```python
from build123d import *

# Parameters (mm, degrees)
BOSS_EXTRUDE1_DEPTH = 24
SKETCH2_R           = 10
BOSS_EXTRUDE2_DEPTH = 24
CIRPATTERN1_COUNT   = 4
BOSS_EXTRUDE4_START = -38
BOSS_EXTRUDE4_DEPTH = 14
BOSS_EXTRUDE5_DEPTH = 14
CUT_EXTRUDE1_DEPTH  = 102.434708064
FILLET1_R           = 10
FILLET2_R           = 10


with BuildPart() as part:
    # Sketch1 → Boss-Extrude1 (new body)
    with BuildSketch(Plane.YZ):
        with BuildLine():
            Line((81, 12), (81, 26))
            Line((81, 26), (37, 26))
            ThreePointArc((37, 26), (23.509262437, 22.226110771), (13.934874811, 12))
            Line((13.934874811, 12), (-37, 12))
            Line((-37, 12), (-37, -12))
            Line((-37, -12), (13.934874811, -12))
            ThreePointArc((13.934874811, -12), (23.509262437, -22.226110771), (37, -26))
            Line((37, -26), (81, -26))
            Line((81, -26), (81, -12))
            Line((81, -12), (37, -12))
            ThreePointArc((37, -12), (25, 0), (37, 12))
            Line((37, 12), (81, 12))
        make_face()
    extrude(amount=BOSS_EXTRUDE1_DEPTH)

    # Sketch2 → Boss-Extrude2 (add)
    with BuildSketch(Plane.XZ.offset(37)):
        with Locations(Location((12, 0, 0), (0, 0, 270))):
            Circle(SKETCH2_R)
    extrude(amount=BOSS_EXTRUDE2_DEPTH)

    # Sketch3 → Cut-Revolve2 (revolve, cut)
    with BuildSketch(Plane.YZ.offset(24)):
        with BuildLine():
            Line((-37, 12), (-37, 6))
            Line((-37, 6), (-17, 6))
            ThreePointArc((-17, 6), (-12.757359313, 7.757359313), (-11, 12))
            Line((-11, 12), (-37, 12))
        make_face()
    cut_revolve2 = revolve(axis=Axis((24, 13.934874811, 12), (0, 1, 0)), mode=Mode.SUBTRACT)

    # CirPattern1: Cut-Revolve2 ×4 about axis
    cirpattern1_axis = Axis((12, 0, 0), (0, 1, 0))
    for i in range(1, CIRPATTERN1_COUNT):
        add(cut_revolve2.rotate(cirpattern1_axis, i * 360 / CIRPATTERN1_COUNT), mode=Mode.SUBTRACT)

    # Sketch4 → Boss-Extrude4 (add, through all)
    with BuildSketch(Plane.XY.offset(26).offset(BOSS_EXTRUDE4_START)):
        with BuildLine():
            Line((24, 61), (24, 45))
            ThreePointArc((24, 45), (29.88854382, 52.05572809), (32, 61))
            ThreePointArc((32, 61), (29.88854382, 69.94427191), (24, 77))
            Line((24, 77), (24, 61))
        make_face()
        with BuildLine():
            Line((0, 45), (0, 61))
            Line((0, 61), (0, 77))
            ThreePointArc((0, 77), (-8, 61), (0, 45))
        make_face()
    extrude(amount=-BOSS_EXTRUDE4_DEPTH)

    # Sketch4<3> → Boss-Extrude5 (add)
    with BuildSketch(Plane.XY.offset(26)):
        with BuildLine():
            Line((24, 61), (24, 45))
            ThreePointArc((24, 45), (29.88854382, 52.05572809), (32, 61))
            ThreePointArc((32, 61), (29.88854382, 69.94427191), (24, 77))
            Line((24, 77), (24, 61))
        make_face()
        with BuildLine():
            Line((0, 45), (0, 61))
            Line((0, 61), (0, 77))
            ThreePointArc((0, 77), (-8, 61), (0, 45))
        make_face()
    extrude(amount=-BOSS_EXTRUDE5_DEPTH)

    # Sketch4<4> → Cut-Extrude1 (cut, through all)
    with BuildSketch(Plane.XY.offset(26)):
        with BuildLine():
            Line((24, 81), (12, 81))
            ThreePointArc((12, 81), (18.32455532, 79.973665961), (24, 77))
            Line((24, 77), (24, 81))
        make_face()
        with BuildLine():
            Line((0, 81), (0, 77))
            ThreePointArc((0, 77), (5.67544468, 79.973665961), (12, 81))
            Line((12, 81), (0, 81))
        make_face()
        with BuildLine():
            ThreePointArc((22, 61), (12, 71), (2, 61))
            Line((2, 61), (12, 61))
            Line((12, 61), (22, 61))
        make_face()
        with BuildLine():
            Line((12, 61), (2, 61))
            ThreePointArc((2, 61), (12, 51), (22, 61))
            Line((22, 61), (12, 61))
        make_face()
    extrude(amount=-CUT_EXTRUDE1_DEPTH, mode=Mode.SUBTRACT)

    # Fillet1
    fillet1_edges = [part.edges().sort_by_distance(p)[0] for p in [
        (24, 45, -19),
        (0, 45, -19),
        (24, 45, 19),
        (0, 45, 19),
    ]]
    fillet(fillet1_edges, radius=FILLET1_R)

    # Fillet2
    fillet2_edges = [part.edges().sort_by_distance(p)[0] for p in [
        (12, 13.934874811, -12),
        (12, 13.934874811, 12),
    ]]
    fillet(fillet2_edges, radius=FILLET2_R)


solid = part.part
```
Part model, mm, in its own coordinate system. A direction names the side the tool comes from. Coordinates: 2 decimals unless noted, no trailing zeros. Order: outer loops, then holes, each group sorted by start corner. A loop starts at its lowest first (then second) coordinate and runs counter-clockwise, first axis right, second up. Notation, with made-up numbers: (51.5, 49.25) - (67.5, 49.25) arc R19 ccw to (67.5, 78.25) - close; hole circle Ø2 at (59.25, 3.5). An arc over 180 degrees is marked (long way). Return JSON: item names as keys, results as strings. Group by question number.
Item 1: Cut at D-D (z = 0). List the corners of the cut face in (x, y).
Item 2: Which spindle directions (+Z, -Z, +X, -X, +Y, -Y) get a long thin tool onto all of the face, cutting with end or side? Do faces 1 (the face through (4.196, -26.86, -7.711)), 2 (the face through (12, -10, -12)), 3 (the face through (24, 10, 0)), 4 (the face through (4.289, -26.86, 7.804)), 5 (the face through (12, 49, 12)). Say none if no direction does.
Item 3: Cut at B-B (x = 15.5). List the corners of the cut face in (y, z), plus the area to 3 significant figures.
Item 4: Pull direction Y, two halves, no side cores. Call faces 6 (the face through (14.17, 70.76, 19.1)), 7 (the face through (19.804, -26.86, 7.711)), 8 (the face through (11.832, 25.685, 23.409)): pulls with the +Y half, pulls with the -Y half, needs draft (parallel to the pull), parting line crosses it, or undercut.
Item 5: Pin check, flat tips, straight feed: pin 1 (6 mm diameter, centred on x = 3.5, y = -44.5, fed in from +Z); pin 2 (5 mm diameter, centred on x = -2, z = -2.5, fed in from +Y); pin 3 (1.5 mm diameter, centred on x = 13, z = -15, fed in from +Y). Stop position of each tip, or through.
Item 6: Cut at A-A (y = 61). List the corners of the cut face in (x, z).
Item 7: Cut at C-C (z = 17.5). List the corners of the cut face in (x, y).
Item 8: Drill centre lines: probe 1 along X at (y, z) = (61, -18); probe 2 along Z at (x, y) = (-4, 70.5); probe 3 along Y at (x, z) = (12, 21.25). Where is each one in solid material? Low to high. Write a range as from..to.
Check values:
{
 "1": {"outline": "(0, -37) - (2, -37) - (2, -61) - (22, -61) - (22, -37) - (24, -37) - (24, 25) - (0, 25) - close"},
 "2": {"face 1": "-Z, -X, -Y", "face 2": "-Z, +X, -X, -Y", "face 3": "+Z, -Z, +X, -Y", "face 4": "+Z, -X, -Y", "face 5": "+X, -X, +Y"},
 "3": {"outline": "(-61, -9.37) - (-37, -9.37) - (-37, -12) - (8.5, -12) arc R10 cw to (16.42, -15.89) arc R26 ccw to (37, -26) - (51.63, -26) - (51.63, -12) - (37, -12) arc R12 cw to (37, 12) - (51.63, 12) - (51.63, 26) - (37, 26) arc R26 ccw to (16.42, 15.89) arc R10 cw to (8.5, 12) - (-37, 12) - (-37, 9.37) - (-61, 9.37) - close; (70.37, -26) - (80.69, -26) - (80.69, -12) - (70.37, -12) - close; (70.37, 12) - (80.69, 12) - (80.69, 26) - (70.37, 26) - close", "area": "3,170 mm2"},
 "4": {"face 6": "undercut", "face 7": "needs draft", "face 8": "pulls with the -Y half"},
 "5": {"pin 1": "stops at z = 8.35", "pin 2": "stops at y = 25.69", "pin 3": "stops at y = 81"},
 "6": {"outline": "(-8, -26) - (2, -26) - (2, -12) - (-8, -12) - close; (-8, 12) - (2, 12) - (2, 26) - (-8, 26) - close; (22, -26) - (32, -26) - (32, -12) - (22, -12) - close; (22, 12) - (32, 12) - (32, 26) - (22, 26) - close"},
 "7": {"outline": "(-2.67, 47.4) arc R10 cw to (0, 40.6) - (0, 17.77) - (24, 17.77) - (24, 40.6) arc R10 cw to (26.67, 47.4) arc R20 ccw (long way) to start; hole circle Ø20 at (12, 61)"},
 "8": {"probe 1": "x = -8..2, 22..32", "probe 2": "z = -26..-12, 12..26", "probe 3": "y = 22.02..51, 71..81"}
}
